```python
from build123d import *

# Parameters (mm, degrees)
SKETCH1_R           = 3.7
BOSS_EXTRUDE1_DEPTH = 3
SKETCH2_W           = 17.5
SKETCH2_H           = 4.507827608
BOSS_EXTRUDE2_DEPTH = 20
SKETCH3_R           = 2.375
BOSS_EXTRUDE3_DEPTH = 20
CUT_EXTRUDE1_REACH  = 71.092
SKETCH6_W           = 3
SKETCH6_H           = 20
BOSS_EXTRUDE4_DEPTH = 23
CUT_EXTRUDE2_REACH  = 79.931
SKETCH7_R           = 3.5
CUT_EXTRUDE3_REACH  = 68.934
SKETCH8_R           = 3.5


with BuildPart() as part:
    # Sketch1 → Boss-Extrude1 (new body)
    with BuildSketch(Plane(origin=(0, 0, 0), x_dir=(1, 0, 0), z_dir=(0, 1, 0))):
        with BuildLine():
            Line((-32, 0), (-32, 40))
            ThreePointArc((-32, 40), (-28.485281374, 48.485281374), (-20, 52))
            Line((-20, 52), (20, 52))
            ThreePointArc((20, 52), (28.485281374, 48.485281374), (32, 40))
            Line((32, 40), (32, 0))
            ThreePointArc((32, 0), (28.485281374, -8.485281374), (20, -12))
            Line((20, -12), (-20, -12))
            ThreePointArc((-20, -12), (-28.485281374, -8.485281374), (-32, 0))
        make_face()
        with Locations(Location((20, 0, 0), (0, 0, 270))):
            Circle(SKETCH1_R, mode=Mode.SUBTRACT)
        with Locations(Location((-20, 0, 0), (0, 0, 270))):
            Circle(SKETCH1_R, mode=Mode.SUBTRACT)
        with Locations(Location((0, 40, 0), (0, 0, 270))):
            Circle(SKETCH1_R, mode=Mode.SUBTRACT)
    extrude(amount=BOSS_EXTRUDE1_DEPTH)

    # Sketch2 → Boss-Extrude2 (add)
    with BuildSketch(Plane(origin=(0, 3, 0), x_dir=(1, 0, 0), z_dir=(0, 1, 0))):
        with Locations((19.25, 35.622787036)):
            Rectangle(SKETCH2_W, SKETCH2_H)
        with Locations((-19.25, 35.622787036)):
            Rectangle(SKETCH2_W, SKETCH2_H)
    extrude(amount=BOSS_EXTRUDE2_DEPTH)

    # Sketch3 → Boss-Extrude3 (add)
    with BuildSketch(Plane(origin=(0, 0, -37.87670084), x_dir=(-1, 0, 0), z_dir=(0, 0, -1))):
        with Locations(Location((-19.25, 13, 0), (0, 0, 180))):
            Circle(SKETCH3_R)
        with Locations(Location((19.25, 13, 0), (0, 0, 180))):
            Circle(SKETCH3_R)
    extrude(amount=BOSS_EXTRUDE3_DEPTH)

    # Sketch5 → Cut-Extrude1 (cut, up to next)
    with BuildSketch(Plane(origin=(0, 3, 0), x_dir=(1, 0, 0), z_dir=(0, 1, 0)), mode=Mode.PRIVATE) as cut_extrude1_sk1:
        with BuildLine():
            Line((-32, 37.87670084), (-10.5, 37.87670084))
            Line((-10.5, 37.87670084), (-10.5, 52))
            Line((-10.5, 52), (-20, 52))
            ThreePointArc((-20, 52), (-28.485281374, 48.485281374), (-32, 40))
            Line((-32, 40), (-32, 37.87670084))
        make_face()
    cut_extrude1_tool1 = extrude(cut_extrude1_sk1.sketch, amount=-CUT_EXTRUDE1_REACH, mode=Mode.PRIVATE) & part.part
    # Sketch5 → Cut-Extrude1 (cut, up to next)
    with BuildSketch(Plane(origin=(0, 3, 0), x_dir=(1, 0, 0), z_dir=(0, 1, 0)), mode=Mode.PRIVATE) as cut_extrude1_sk2:
        with BuildLine():
            Line((32, 37.87670084), (10.5, 37.87670084))
            Line((10.5, 37.87670084), (10.5, 52))
            Line((10.5, 52), (20, 52))
            ThreePointArc((20, 52), (28.485281374, 48.485281374), (32, 40))
            Line((32, 40), (32, 37.87670084))
        make_face()
    cut_extrude1_tool2 = extrude(cut_extrude1_sk2.sketch, amount=-CUT_EXTRUDE1_REACH, mode=Mode.PRIVATE) & part.part
    add(cut_extrude1_tool1.solids().sort_by_distance((-20.335708, 3, -44.441952))[0], mode=Mode.SUBTRACT)
    add(cut_extrude1_tool2.solids().sort_by_distance((20.335708, 3, -44.441952))[0], mode=Mode.SUBTRACT)

    # Sketch6 → Boss-Extrude4 (add)
    with BuildSketch(Plane(origin=(0, 3, 0), x_dir=(1, 0, 0), z_dir=(0, 1, 0))):
        with Locations((-11.75, 18.15)):
            Rectangle(SKETCH6_W, SKETCH6_H)
        Polygon((13.25, 8.15), (10.25, 8.15), (-10.25, 8.15), (-13.25, 8.15), (-13.25, 5.15), (13.25, 5.15), align=None)
        with Locations((11.75, 18.15)):
            Rectangle(SKETCH6_W, SKETCH6_H)
    extrude(amount=BOSS_EXTRUDE4_DEPTH)

    # Cut-Extrude2: up to this face of the body (flat: up to its plane)
    cut_extrude2_end = Plane(part.part.faces().sort_by_distance((13.25, 14.5, -16.65))[0])
    # Sketch7 → Cut-Extrude2 (cut, up to the picked face)
    with BuildSketch(Plane.ZY.offset(13.25), mode=Mode.PRIVATE) as cut_extrude2_sk1:
        with Locations((-18.15, 14.5)):
            Circle(SKETCH7_R)
    cut_extrude2_tool1 = split(extrude(cut_extrude2_sk1.sketch, amount=-CUT_EXTRUDE2_REACH, mode=Mode.PRIVATE), bisect_by=cut_extrude2_end, keep=Keep.BOTH, mode=Mode.PRIVATE)
    add(cut_extrude2_tool1.solids().sort_by(Axis((-13.25, 14.5, -18.15), (1, 0, 0)))[0], mode=Mode.SUBTRACT)

    # Sketch8 → Cut-Extrude3 (cut, up to next)
    with BuildSketch(Plane.XY.offset(-5.15), mode=Mode.PRIVATE) as cut_extrude3_sk1:
        with Locations((0, 14.5)):
            Circle(SKETCH8_R)
    cut_extrude3_tool1 = extrude(cut_extrude3_sk1.sketch, amount=-CUT_EXTRUDE3_REACH, mode=Mode.PRIVATE) & part.part
    add(cut_extrude3_tool1.solids().sort_by_distance((0, 14.5, -5.15))[0], mode=Mode.SUBTRACT)


solid = part.part
```
Here's how the part is built. I have some questions about the finished solid (model axes, mm). A direction names the side the tool comes from. Round coordinates to 2 decimals unless told otherwise and drop trailing zeros. Loops run counter-clockwise (first coordinate to the right, second up) from the corner with the lowest first, then second, coordinate; pieces in that order, holes last. Notation, with made-up numbers: (88.5, 61.5) -> (129.5, 61.5) arc R31 cw to (129.5, 91.5) -> close; hole circle Ø2 at (-12, -38). An arc over 180 degrees is marked (long way). Answer as CSV lines item,"result". Start each with the question number.
1. For faces 4 (the face through (3, 17, -5.15)), 5 (the face through (-10.5, 2, -45)), 6 (the face through (-12, 14, -28.15)), 7 (the face through (10.25, 14, -14)), 8 (the face through (16.72, 1.48, 1.71)), which set-ups out of +Z, -Z, +X, -X, +Y, -Y let a thin tool reach every point of the face, with its end or its side?
2. I'm going to push flat-ended pins straight in: P1, Ø12, axis at y = 16.5, z = -44, coming from the +X side (3 decimals); P2, Ø4, axis at x = -22, y = 18, coming from the +Z side; P3, Ø10, axis at y = 19, z = -20.5, coming from the -X side; P4, Ø1, axis at x = 19, z = -21.5, coming from the -Y side. Where does each tip first touch, or does it pass through?
3. I need wall thicknesses on probe 1 along X at (y, z) = (2.35, 0); probe 2 along X at (y, z) = (2.1, -40); probe 3 along X at (y, z) = (6, -22). Which ranges of each line are inside material? Lowest first, please. Write a range as from..to.
4. Imagine slicing it at C-C on z = -18.15. Write out the boundary of the cut face in (x, y), plus the area to 3 significant figures.
5. Imagine slicing it at D-D on x = -18. Write out the boundary of the cut face in (y, z).
6. Imagine slicing it at B-B on y = 5. Write out the boundary of the cut face in (x, z), plus the area to 3 significant figures.
7. Imagine slicing it at A-A on z = -40. Write out the boundary of the cut face in (x, y) (3 decimals), plus the area to 3 significant figures.
8. If we mould it in two halves opening along Z, with no side actions, what happens to faces 1 (the face through (28.58, 1.48, 8.39)), 2 (the face through (-32, 1, -19)), 3 (the face through (12, 14, -28.15))? For each: pulls with the +Z half, pulls with the -Z half, needs draft (parallel to the pull), parting line crosses it, or undercut.
Solution:
1,face 4,"+Z, +X, -X, +Y"
1,face 5,"-Z, -X, +Y, -Y"
1,face 6,"+X, -X, +Y"
1,face 7,"-Z, +Y"
1,face 8,"+Y, -Y"
2,P1,"x = 21.625"
2,P2,"z = -33.37"
2,P3,"x = -13.25"
2,P4,"y = 0"
3,probe 1,"-32..-23.7, -16.3..16.3, 23.7..32"
3,probe 2,"-10.5..-3.7, 3.7..10.5"
3,probe 3,"-13.25..-10.25, 10.25..13.25"
4,outline,"(-32, 0) -> (32, 0) -> (32, 3) -> (13.25, 3) -> (13.25, 11) -> (10.25, 11) -> (10.25, 3) -> (-10.25, 3) -> (-10.25, 11) -> (-13.25, 11) -> (-13.25, 3) -> (-32, 3) -> close; (-13.25, 18) -> (-10.25, 18) -> (-10.25, 26) -> (-13.25, 26) -> close; (10.25, 18) -> (13.25, 18) -> (13.25, 26) -> (10.25, 26) -> close"
4,area,"288 mm²"
5,outline,"(0, -37.88) -> (10.98, -37.88) -> (10.98, -57.88) -> (15.02, -57.88) -> (15.02, -37.88) -> (23, -37.88) -> (23, -33.37) -> (3, -33.37) -> (3, -3.11) -> (0, -3.11) -> close; (0, 3.11) -> (3, 3.11) -> (3, 12) -> (0, 12) -> close"
6,outline,"(-28, -37.88) -> (-10.5, -37.88) -> (-10.5, -33.37) -> (-28, -33.37) -> close; (-13.25, -28.15) -> (-10.25, -28.15) -> (-10.25, -8.15) -> (10.25, -8.15) -> (10.25, -28.15) -> (13.25, -28.15) -> (13.25, -5.15) -> (-13.25, -5.15) -> close; (10.5, -37.88) -> (28, -37.88) -> (28, -33.37) -> (10.5, -33.37) -> close"
6,area,"357 mm²"
7,outline,"circle Ø4.75 at (-19.25, 13); (-10.5, 0) -> (-3.7, 0) -> (-3.7, 3) -> (-10.5, 3) -> close; (3.7, 0) -> (10.5, 0) -> (10.5, 3) -> (3.7, 3) -> close; circle Ø4.75 at (19.25, 13)"
7,area,"76.2 mm²"
8,face 1,"pulls with the +Z half"
8,face 2,"needs draft"
8,face 3,"undercut"
